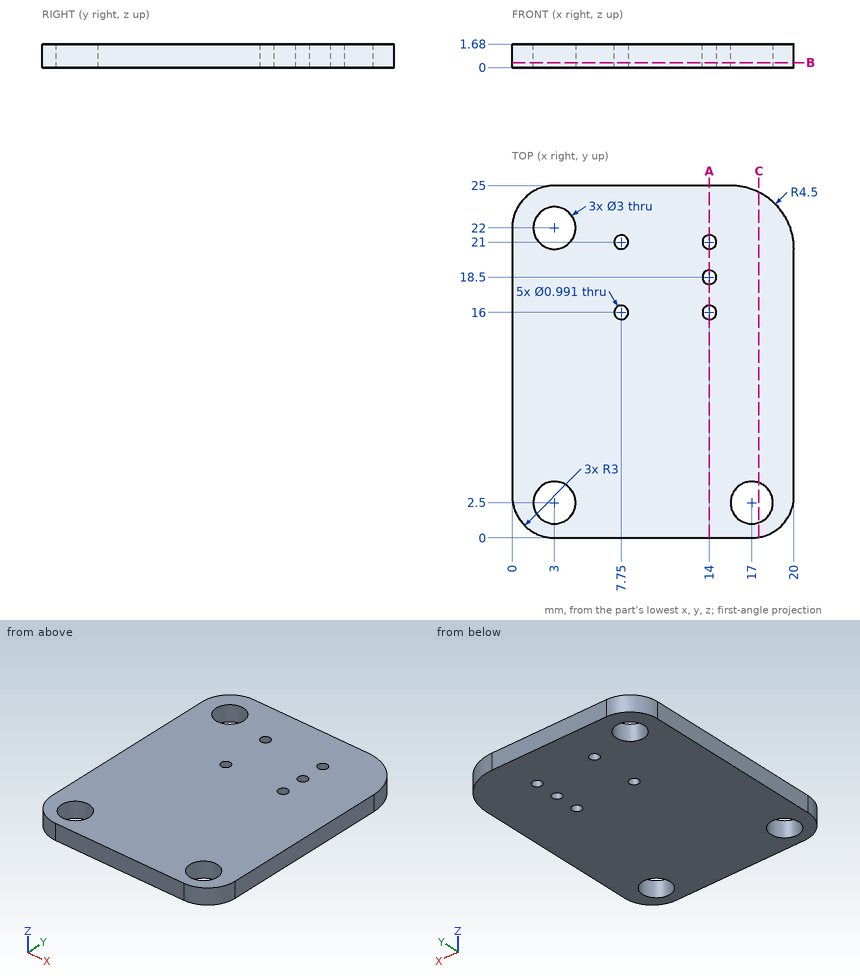
Drawing for the job (mm, zero at the part's lowest x, y, z). Round coordinates to 2 decimals unless told otherwise and drop trailing zeros. Write each loop counter-clockwise with the first axis right and the second up, starting at its lowest first coordinate (ties: lowest second). Pieces come first, ordered by that corner, then holes. Notation, with made-up numbers: M 8.25,31.5 L 16.25,31.5 A24 cw 16.25,58.5 Z; hole C 81,75.5 d8. An arc over 180 degrees is marked long. One line per question, with ' | ' between items.
1. Pin check, flat tip, straight feed: pin 1 Ø1.8 at (x, y) = (3, 2.5) entering from -Z. Stop position of the tip, or through.
Working result:
pin 1: through
2. Probe L1, parallel to Y at x = 14, z = 1.35 (1 decimal); L2, parallel to Y at x = 3, z = 1.15; L3, parallel to X at y = 16, z = 1.1 (1 decimal). List the from-to ranges inside material, lowest first. Write a range as from..to.
Working result:
L1: 0..15.5, 16.5..18, 19..20.5, 21.5..25 | L2: 0..1, 4..20.5, 23.5..25 | L3: 0..7.3, 8.2..13.5, 14.5..20
3. Cut at A-A on x = 14. Write the cut outline in (y, z) (1 decimal).
Working result:
outline: M 0,0 L 15.5,0 L 15.5,1.7 L 0,1.7 Z; M 16.5,0 L 18,0 L 18,1.7 L 16.5,1.7 Z; M 19,0 L 20.5,0 L 20.5,1.7 L 19,1.7 Z; M 21.5,0 L 25,0 L 25,1.7 L 21.5,1.7 Z
4. Cut at B-B on z = 0.35. Count the separate pieces of the cut face and the enclosed holes in it, and give its area (3 significant figures).
Working result:
separate pieces: 1 | enclosed holes: 8 | area: 465 mm2
5. Cut at C-C on x = 17.5. Write the cut outline in (y, z) (1 decimal).
Working result:
outline: M 0,0 L 1.1,0 L 1.1,1.7 L 0,1.7 Z; M 3.9,0 L 24.5,0 L 24.5,1.7 L 3.9,1.7 Z
